```python
from build123d import *

# Parameters (mm, degrees)
F0_W     = 36.83
F0_H     = 76.2
F1_DEPTH = 3.81
F2_W     = 8.89
F2_H     = 3.81
F3_DEPTH = 3.81
F4_W     = 8.89
F4_H     = 3.81
F5_DEPTH = 3.81


with BuildPart() as f1:
    # F0 (on Front) → F1 (new body)
    with BuildSketch(Plane.XZ):
        Polygon((-88.9, -66.0091239631), (0, -66.0091239631), (88.9, -66.0091239631), (88.9, 22.8908760369), (0, 92.7408760369), (-88.9, 22.8908760369), align=None)
        with Locations((-60.325, -15.2091239631)):
            Rectangle(F0_W, F0_H, mode=Mode.SUBTRACT)
        with Locations((60.325, -15.2091239631)):
            Rectangle(F0_W, F0_H, mode=Mode.SUBTRACT)
    extrude(amount=F1_DEPTH)

    # F2 (on face) → F3 (cut)
    with BuildSketch(Plane(origin=(-45.0539271599, 0, 57.3413618398), x_dir=(0.7863183388, 0, 0.6178215519), z_dir=(-0.6178215519, 0, 0.7863183388))):
        with Locations((-14.4576880394, -1.905)):
            Rectangle(F2_W, F2_H)
        with Locations((23.6423119606, -1.905)):
            Rectangle(F2_W, F2_H)
        with Locations((42.6923119606, -1.905)):
            Rectangle(F2_W, F2_H)
        with Locations((4.5923119606, -1.905)):
            Rectangle(F2_W, F2_H)
    extrude(amount=-F3_DEPTH, mode=Mode.SUBTRACT)

    # F4 (on face) → F5 (cut)
    with BuildSketch(Plane(origin=(45.0539271599, 0, 57.3413618398), x_dir=(0.7863183388, 0, -0.6178215519), z_dir=(0.6178215519, 0, 0.7863183388))):
        with Locations((-42.6923119606, -1.905)):
            Rectangle(F4_W, F4_H)
        with Locations((-23.6423119606, -1.905)):
            Rectangle(F4_W, F4_H)
        with Locations((-4.5923119606, -1.905)):
            Rectangle(F4_W, F4_H)
        with Locations((14.4576880394, -1.905)):
            Rectangle(F4_W, F4_H)
    extrude(amount=-F5_DEPTH, mode=Mode.SUBTRACT)


solid = f1.part
```
Geometry check sheet. Reference: the model listing, model coordinates, mm. A direction names the side the tool comes from. Round coordinates to 2 decimals unless told otherwise and drop trailing zeros. Order: outer loops, then holes, each group sorted by start corner. A loop starts at its lowest first (then second) coordinate and runs counter-clockwise, first axis right, second up. Notation, with made-up numbers: (24.5, -22) - (68.5, -22) arc R6 ccw to (68.5, -18) - close; hole circle Ø10 at (59.25, -19). An arc over 180 degrees is marked (long way). Use a Markdown table: item, result. Add a question column.
(1) Sectioned sample at C-C, the plane y = -0.95. Count the separate pieces of the cut face and the enclosed holes in it, and give its area (3 significant figures).
(2) Sectioned sample at B-B, the plane x = 72.5. Enter the section's corners in (y, z), and give its area (3 significant figures).
(3) Release check for a two-part mould opening along X. For faces 3 (the flat face through (-18.918, -1.878, 77.877)), 4 (the flat face through (-1, -2, -66.009)), 5 (the flat face through (60, -2, -53.309)), 6 (the flat face through (88.9, -2, -22)) record: pulls with the +X half, pulls with the -X half, needs draft (parallel to the pull), parting line crosses it, or undercut.
(4) Depth check by flat-ended pin: pin 1 (1.9 mm diameter, centred on x = -63.5, y = -1.5, fed in from +Z). Enter the tip coordinate at first touch or a pass-through.
(5) Tool access check on faces 1 (the flat face through (9.08, -1.88, 80.76)), 2 (the flat face through (-3.939, -1.878, 89.646)). Record the directions out of +Z, -Z, +X, -X, +Y, -Y that give a thin tool (end or side, any length) a straight path to the whole face; none if there is none.
(6) Material ranges on line 1 along X through (y, z) = (-1.2, -42); line 2 along Z through (x, y) = (-37, -3); line 3 along Z through (x, y) = (43.5, -3.2), recorded low to high. Write a range as [from, to].
(7) Sectioned sample at A-A, the plane z = -25. Enter the section's corners in (x, y), and give its area (3 significant figures).
Answers below:
| question | item | result |
|---|---|---|
| 1 | separate pieces | 1 |
| 1 | enclosed holes | 2 |
| 1 | area | 16,100 mm² |
| 2 | outline | (-3.81, -66.01) - (0, -66.01) - (0, -53.31) - (-3.81, -53.31) - close; (-3.81, 22.89) - (0, 22.89) - (0, 35.78) - (-3.81, 35.78) - close |
| 2 | area | 97.5 mm² |
| 3 | face 3 | pulls with the -X half |
| 3 | face 4 | needs draft |
| 3 | face 5 | undercut |
| 3 | face 6 | pulls with the +X half |
| 4 | pin 1 | z = 43.59 |
| 5 | face 1 | +Y, -Y |
| 5 | face 2 | +Z, -X, +Y, -Y |
| 6 | line 1 | [-88.9, -78.74], [-41.91, 41.91], [78.74, 88.9] |
| 6 | line 2 | [-66.01, 58.82], [61.72, 63.67] |
| 6 | line 3 | [-66.01, -53.31], [22.89, 55.6] |
| 7 | outline | (-88.9, -3.81) - (-78.74, -3.81) - (-78.74, 0) - (-88.9, 0) - close; (-41.91, -3.81) - (41.91, -3.81) - (41.91, 0) - (-41.91, 0) - close; (78.74, -3.81) - (88.9, -3.81) - (88.9, 0) - (78.74, 0) - close |
| 7 | area | 397 mm² |
